The listing builds one solid part. Answer for the finished solid, in the listing's coordinates (mm). A direction names the side the tool comes from. Round coordinates to 2 decimals unless told otherwise and drop trailing zeros. Write each loop counter-clockwise with the first axis right and the second up, starting at its lowest first coordinate (ties: lowest second). Pieces come first, ordered by that corner, then holes.
Item 1: Each of these flat-tipped pins is pushed along its axis until it touches: pin 1 (2 mm diameter, centred on y = 5.5, z = -5.5, fed in from +X) (3 decimals); pin 2 (4 mm diameter, centred on x = 5, z = -5, fed in from +Y); pin 3 (1 mm diameter, centred on y = 7.5, z = -1, fed in from +X); pin 4 (2 mm diameter, centred on x = 29, z = -3.5, fed in from -Y). Where does it stop, or does it pass through?
Item 2: Find section D-D on x = 37. Give the vertices of the cut face in (y, z), then the cut area to 3 significant figures.
Item 3: Find section A-A on z = -5. Give the vertices of the cut face in (x, y), then the cut area to 3 significant figures.
Item 4: For a pull along Z with two mould halves and no side action, classify faces 1 (the face through (69.14, 1.52, -9.1)), 2 (the face through (66.669, 1.479, -5.526)), 3 (the face through (0, 1, -5)) as +Z half, -Z half, draft (parallel to the pull), parting line (faces both ways), or undercut.
Item 5: Find section B-B on x = 65. Give the vertices of the cut face in (y, z), then the cut area to 3 significant figures.
Item 6: Find section C-C on y = 1.75. Give the vertices of the cut face in (x, z), then the cut area to 3 significant figures.
Item 7: Find the intervals of material crossed by probe 1 along X at (y, z) = (1.75, -5); probe 2 along Z at (x, y) = (65, 1.25); probe 3 along Y at (x, z) = (38.5, -7.25), in increasing order.
Item 8: A tool of negligible diameter and unlimited length cuts with its end or side. For faces 4 (the face through (16, 6, -5)), 5 (the face through (3, 3, -5)), 6 (the face through (67, 3, -4)), from which of +Z, -Z, +X, -X, +Y, -Y can it reach the whole face along a straight path? Write none if from no direction.
```python
from build123d import *

# Parameters (mm, degrees)
SKETCH1_W           = 70
SKETCH1_H           = 10
SKETCH1_R           = 1.75
BOSS_EXTRUDE1_DEPTH = 3
EXTRUDE_THIN1_DEPTH = 10
CUT_EXTRUDE1_REACH  = 12
FILLET1_R           = 3
FILLET2_R           = 1


with BuildPart() as part:
    # Sketch1 → Boss-Extrude1 (new body)
    with BuildSketch(Plane(origin=(0, 0, 0), x_dir=(1, 0, 0), z_dir=(0, 1, 0))):
        with Locations((35, 5)):
            Rectangle(SKETCH1_W, SKETCH1_H)
        with Locations((5, 5)):
            Circle(SKETCH1_R, mode=Mode.SUBTRACT)
        with Locations((65, 5)):
            Circle(SKETCH1_R, mode=Mode.SUBTRACT)
    extrude(amount=BOSS_EXTRUDE1_DEPTH)

    # Sketch2 → Extrude-Thin1 (add)
    with BuildSketch(Plane.XY):
        Polygon((10, 3), (16, 11), (54, 11), (60, 3), align=None)
        Polygon((16, 6), (17.5, 8), (52.5, 8), (54, 6), align=None, mode=Mode.SUBTRACT)
    extrude(amount=-EXTRUDE_THIN1_DEPTH)

    # Sketch3 → Cut-Extrude1 (cut, up to next)
    with BuildSketch(Plane.XY, mode=Mode.PRIVATE) as cut_extrude1_sk1:
        Polygon((16, 6), (13.75, 3), (56.25, 3), (54, 6), align=None)
    cut_extrude1_tool1 = extrude(cut_extrude1_sk1.sketch, amount=-CUT_EXTRUDE1_REACH, mode=Mode.PRIVATE) & part.part
    add(cut_extrude1_tool1.solids().sort_by_distance((35, 4.47205, 0))[0], mode=Mode.SUBTRACT)

    # Fillet1
    fillet1_edges = [part.edges().sort_by_distance(p)[0] for p in [
        (54, 11, -5),
        (16, 11, -5),
        (10, 3, -5),
        (60, 3, -5),
        (52.5, 8, -5),
        (17.5, 8, -5),
        (0, 1.5, -10),
        (70, 1.5, -10),
        (70, 1.5, 0),
        (0, 1.5, 0),
    ]]
    fillet(fillet1_edges, radius=FILLET1_R)

    # Fillet2
    fillet2_edges = [part.edges().sort_by_distance(p)[0] for p in [
        (56.25, 3, -5),
        (13.75, 3, -5),
    ]]
    fillet(fillet2_edges, radius=FILLET2_R)


solid = part.part
```
Check values:
1. pin 1: stops at x = 58.875
1. pin 2: stops at y = 3
1. pin 3: stops at x = 57
1. pin 4: stops at y = 0
2. outline: (0, -10) - (3, -10) - (3, 0) - (0, 0) - close; (8, -10) - (11, -10) - (11, 0) - (8, 0) - close
2. area: 60.0 mm2
3. outline: (0, 0) - (3.25, 0) - (3.25, 3) - (0, 3) - close; (6.75, 0) - (63.25, 0) - (63.25, 3) - (61.5, 3) arc R3 cw to (59.1, 4.2) - (54.9, 9.8) arc R3 ccw to (52.5, 11) - (17.5, 11) arc R3 ccw to (15.1, 9.8) - (10.9, 4.2) arc R3 cw to (8.5, 3) - (6.75, 3) - close; (66.75, 0) - (70, 0) - (70, 3) - (66.75, 3) - close; hole (14.95, 4.6) arc R1 ccw to (15.75, 3) - (54.25, 3) arc R1 ccw to (55.05, 4.6) - (53.4, 6.8) arc R3 ccw to (51, 8) - (19, 8) arc R3 ccw to (16.6, 6.8) - close
3. area: 350 mm2
4. face 1: -Z half
4. face 2: undercut
4. face 3: draft
5. outline: (0, -10) - (3, -10) - (3, -6.75) - (0, -6.75) - close; (0, -3.25) - (3, -3.25) - (3, 0) - (0, 0) - close
5. area: 19.5 mm2
6. outline: (0, -7) arc R3 ccw to (3, -10) - (67, -10) arc R3 ccw to (70, -7) - (70, -3) arc R3 ccw to (67, 0) - (3, 0) arc R3 ccw to (0, -3) - close; hole circle Ø3.5 at (5, -5); hole circle Ø3.5 at (65, -5)
6. area: 673 mm2
7. probe 1: x = 0 to 3.25, 6.75 to 63.25, 66.75 to 70
7. probe 2: z = -10 to -6.75, -3.25 to 0
7. probe 3: y = 0 to 3, 8 to 11
8. face 4: +Z, -Z
8. face 5: +Z, -Z, -X, +Y
8. face 6: +Z, -Z, +X, +Y
